from build123d import *

# Parameters (mm, degrees)
F1_DEPTH = 100
F2_R     = 3.5
F3_DEPTH = 25
F4_R     = 1


with BuildPart() as f1:
    # F0 (on Front) → F1 (new body, symmetric)
    with BuildSketch(Plane.XZ):
        with BuildLine():
            Line((11.7, 7.5), (0, 7.5))
            Line((0, 7.5), (-11.7, 7.5))
            ThreePointArc((-11.7, 7.5), (-12.9727922061, 6.9727922061), (-13.5, 5.7))
            Line((-13.5, 5.7), (-13.5, 1.8))
            ThreePointArc((-13.5, 1.8), (-13.7343145751, 1.2343145751), (-14.3, 1))
            Line((-14.3, 1), (-17.5, 1))
            Line((-17.5, 1), (-17.5, 0))
            Line((-17.5, 0), (-14.3, 0))
            ThreePointArc((-14.3, 0), (-13.0272077939, 0.5272077939), (-12.5, 1.8))
            Line((-12.5, 1.8), (-12.5, 5.7))
            ThreePointArc((-12.5, 5.7), (-12.2656854249, 6.2656854249), (-11.7, 6.5))
            Line((-11.7, 6.5), (0, 6.5))
            Line((0, 6.5), (11.7, 6.5))
            ThreePointArc((11.7, 6.5), (12.2656854249, 6.2656854249), (12.5, 5.7))
            Line((12.5, 5.7), (12.5, 1.8))
            ThreePointArc((12.5, 1.8), (13.0272077939, 0.5272077939), (14.3, 0))
            Line((14.3, 0), (17.5, 0))
            Line((17.5, 0), (17.5, 1))
            Line((17.5, 1), (14.3, 1))
            ThreePointArc((14.3, 1), (13.7343145751, 1.2343145751), (13.5, 1.8))
            Line((13.5, 1.8), (13.5, 5.7))
            ThreePointArc((13.5, 5.7), (12.9727922061, 6.9727922061), (11.7, 7.5))
        make_face()
    extrude(amount=F1_DEPTH, both=True)

    # F2 (on face) → F3 (cut)
    with BuildSketch(Plane.XY.offset(7.5)):
        with Locations((0, 53)):
            Circle(F2_R)
        with Locations((0, -53)):
            Circle(F2_R)
    extrude(amount=-F3_DEPTH, mode=Mode.SUBTRACT)

    # F4
    f4_edges = [f1.edges().sort_by_distance(p)[0] for p in [
        (17.5, 100, 0.5),
        (-17.5, 100, 0.5),
        (17.5, -100, 0.5),
        (-17.5, -100, 0.5),
    ]]
    fillet(f4_edges, radius=F4_R)


solid = f1.part
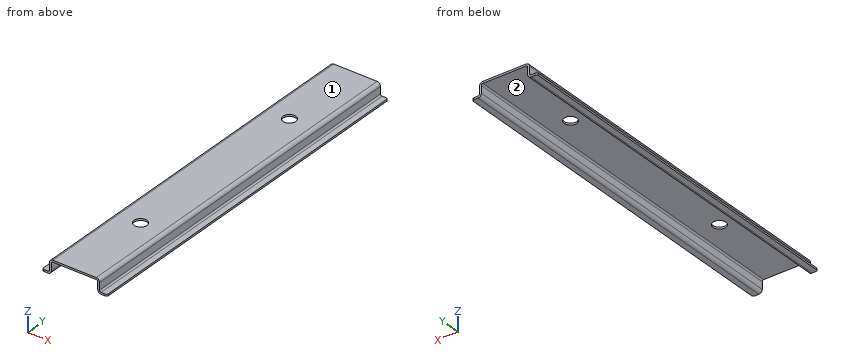
The model under review builds one solid part; all positions refer to its coordinate system, in mm. Face numbers are marked on the shaded views. Coordinates: 2 decimals unless noted, no trailing zeros. Write each loop counter-clockwise with the first axis right and the second up, starting at its lowest first coordinate (ties: lowest second). Pieces come first, ordered by that corner, then holes. Notation, with made-up numbers: (11.25, -17) - (50.25, -17) arc R20 ccw to (50.25, 2) - close; hole circle Ø4 at (3, 87). An arc over 180 degrees is marked (long way). Answer as a JSON object with one key per item and string values. Group by question number.
1. Mouldability with a two-part tool opening along X and no side actions: class the marked faces 1 and 2 as pulls with the +X half, pulls with the -X half, needs draft (parallel to the pull), parting line crosses it, or undercut.
2. Add section A-A (z = 3.5). Give the boundary of the cut face in (x, y), plus the area to 3 significant figures.
3. Add section D-D (y = 13.5). Give the boundary of the cut face in (x, z), plus the area to 3 significant figures.
4. To check wall thickness, follow probe 1 along Y at (x, z) = (0, 6.9); probe 2 along X at (y, z) = (-66, 1.75); probe 3 along Z at (x, y) = (-5.5, -18). State the ranges of each line that lie inside material, in increasing order.
5. Add section B-B (x = 0). Give the boundary of the cut face in (y, z).
6. Clearance check with flat-ended pins moving along their axes: pin 1 Ø1.6 at (x, y) = (-15.5, 11.5) entering from +Z; pin 2 Ø8 at (x, y) = (0, 53) entering from -Z; pin 3 Ø2 at (y, z) = (-9.5, 4.5) entering from -X; pin 4 Ø6.5 at (x, y) = (0, -53) entering from -Z. State where each tip first meets the part, or that it passes through.
7. Add section C-C (y = 53). Give the boundary of the cut face in (x, z).
Findings:
{
 "1": {"face 1": "needs draft", "face 2": "undercut"},
 "2": {"outline": "(-13.5, -100) - (-12.5, -100) - (-12.5, 100) - (-13.5, 100) - close; (12.5, -100) - (13.5, -100) - (13.5, 100) - (12.5, 100) - close", "area": "400 mm²"},
 "3": {"outline": "(-17.5, 0) - (-14.3, 0) arc R1.8 ccw to (-12.5, 1.8) - (-12.5, 5.7) arc R0.8 cw to (-11.7, 6.5) - (11.7, 6.5) arc R0.8 cw to (12.5, 5.7) - (12.5, 1.8) arc R1.8 ccw to (14.3, 0) - (17.5, 0) - (17.5, 1) - (14.3, 1) arc R0.8 cw to (13.5, 1.8) - (13.5, 5.7) arc R1.8 ccw to (11.7, 7.5) - (-11.7, 7.5) arc R1.8 ccw to (-13.5, 5.7) - (-13.5, 1.8) arc R0.8 cw to (-14.3, 1) - (-17.5, 1) - close", "area": "45.8 mm²"},
 "4": {"probe 1": "-100 to -56.5, -49.5 to 49.5, 56.5 to 100", "probe 2": "-13.5 to -12.5, 12.5 to 13.5", "probe 3": "6.5 to 7.5"},
 "5": {"outline": "(-100, 6.5) - (-56.5, 6.5) - (-56.5, 7.5) - (-100, 7.5) - close; (-49.5, 6.5) - (49.5, 6.5) - (49.5, 7.5) - (-49.5, 7.5) - close; (56.5, 6.5) - (100, 6.5) - (100, 7.5) - (56.5, 7.5) - close"},
 "6": {"pin 1": "z = 1", "pin 2": "z = 6.5", "pin 3": "x = -13.5", "pin 4": "through"},
 "7": {"outline": "(-17.5, 0) - (-14.3, 0) arc R1.8 ccw to (-12.5, 1.8) - (-12.5, 5.7) arc R0.8 cw to (-11.7, 6.5) - (-3.5, 6.5) - (-3.5, 7.5) - (-11.7, 7.5) arc R1.8 ccw to (-13.5, 5.7) - (-13.5, 1.8) arc R0.8 cw to (-14.3, 1) - (-17.5, 1) - close; (3.5, 6.5) - (11.7, 6.5) arc R0.8 cw to (12.5, 5.7) - (12.5, 1.8) arc R1.8 ccw to (14.3, 0) - (17.5, 0) - (17.5, 1) - (14.3, 1) arc R0.8 cw to (13.5, 1.8) - (13.5, 5.7) arc R1.8 ccw to (11.7, 7.5) - (3.5, 7.5) - close"}
}
